Verification items for the finished model (mm, model axes). A direction names the side the tool comes from. Round coordinates to 2 decimals unless told otherwise and drop trailing zeros. Order: outer loops, then holes, each group sorted by start corner. A loop starts at its lowest first (then second) coordinate and runs counter-clockwise, first axis right, second up. Notation, with made-up numbers: M -27,32.25 L 11,32.25 A31 cw 11,57.25 Z; hole C 13,-22 d6. An arc over 180 degrees is marked long. Answer as a JSON object with one key per item and string values. Group by question number.
```python
from build123d import *

# Parameters (mm, degrees)
BOSS_EXTRUDE1_DEPTH     = 22.225
CUT_EXTRUDE1_DEPTH      = 15.875
CUT_EXTRUDE2_DEPTH      = 19.05
CUT_EXTRUDE3_DEPTH      = 19.05
CUT_EXTRUDE4_DEPTH      = 15.875
CUT_EXTRUDE5_DEPTH      = 1
CUT_EXTRUDE5_DEPTH_BACK = 45.45
CUT_EXTRUDE6_DEPTH      = 38.1
SKETCH9_R               = 4.75
CUT_EXTRUDE7_DEPTH      = 39.1
CUT_EXTRUDE7_DEPTH_BACK = 7.35
SKETCH10_R              = 5.08
CUT_EXTRUDE8_DEPTH      = 38.1
CUT_EXTRUDE8_DEPTH_BACK = 38.1
SKETCH14_R              = 5.08
CUT_EXTRUDE9_DEPTH      = 88.9


with BuildPart() as part:
    # Sketch1 → Boss-Extrude1 (new body, symmetric)
    with BuildSketch(Plane(origin=(0, 0, 0), x_dir=(1, 0, 0), z_dir=(0, 1, 0))):
        with BuildLine():
            Line((-27.139164257, 167.796683689), (23.215337255, 167.796683689))
            ThreePointArc((23.215337255, 167.796683689), (26.553400644, 166.414012561), (27.936071772, 163.075949172))
            Line((27.936071772, 163.075949172), (27.936071772, 117.442182176))
            Line((27.936071772, 117.442182176), (45.739076513, 99.639177435))
            ThreePointArc((45.739076513, 99.639177435), (52.653298853, 95.043473949), (60.717629895, 93.070271999))
            ThreePointArc((60.717629895, 93.070271999), (72.137749756, 94.950404711), (82.719311408, 99.639177435))
            ThreePointArc((82.719311408, 99.639177435), (99.088819495, 116.502407503), (106.691226482, 138.740499404))
            ThreePointArc((106.691226482, 138.740499404), (107.293250165, 146.399208048), (107.783318293, 154.065894676))
            ThreePointArc((107.783318293, 154.065894676), (108.340552038, 159.17256706), (108.853679748, 164.283859678))
            ThreePointArc((108.853679748, 164.283859678), (109.705429788, 167.387313473), (111.11535679, 170.2802375))
            ThreePointArc((111.11535679, 170.2802375), (113.620556723, 172.466184723), (116.845200472, 173.276162908))
            ThreePointArc((116.845200472, 173.276162908), (120.221594265, 172.465675408), (123.355683212, 170.970880603))
            ThreePointArc((123.355683212, 170.970880603), (128.265134652, 166.745027029), (132.181680011, 161.585451046))
            ThreePointArc((132.181680011, 161.585451046), (138.33428397, 146.199471549), (139.619453347, 129.678840803))
            ThreePointArc((139.619453347, 129.678840803), (136.39277719, 110.641651914), (129.659662699, 92.544934835))
            ThreePointArc((129.659662699, 92.544934835), (120.370646129, 69.036558024), (118.071361376, 43.864293549))
            ThreePointArc((118.071361376, 43.864293549), (122.222572829, 21.498106395), (129.659662699, 0))
            ThreePointArc((129.659662699, 0), (143.398814545, -36.155916163), (153.856513267, -73.393680656))
            ThreePointArc((153.856513267, -73.393680656), (158.275027292, -104.230564471), (157.301620264, -135.367185167))
            ThreePointArc((157.301620264, -135.367185167), (141.975051177, -176.275361149), (106.691226482, -202.032579498))
            ThreePointArc((106.691226482, -202.032579498), (54.098789107, -214.895017574), (0, -217.069367939))
            ThreePointArc((0, -217.069367939), (-54.004742533, -214.862710734), (-106.509687866, -202.032579498))
            ThreePointArc((-106.509687866, -202.032579498), (-141.094553776, -177.085698472), (-156.684587611, -137.394255213))
            ThreePointArc((-156.684587611, -137.394255213), (-153.316704731, -83.564621207), (-134.097306667, -33.170307338))
            ThreePointArc((-134.097306667, -33.170307338), (-118.452837363, -0.106574858), (-106.509687848, 34.466839857))
            ThreePointArc((-106.509687848, 34.466839857), (-104.952609842, 63.858154337), (-111.536110603, 92.544934857))
            ThreePointArc((-111.536110603, 92.544934857), (-124.146260861, 134.317832636), (-132.040568435, 177.232524599))
            ThreePointArc((-132.040568435, 177.232524599), (-132.180605283, 199.253892218), (-127.895077973, 220.854690763))
            ThreePointArc((-127.895077973, 220.854690763), (-123.677084376, 229.09027242), (-117.65146136, 236.112248103))
            ThreePointArc((-117.65146136, 236.112248103), (-112.585214143, 239.486704693), (-106.727388664, 241.141908245))
            ThreePointArc((-106.727388664, 241.141908245), (-101.521494245, 239.144724173), (-99.844107934, 233.82716307))
            Line((-99.844107934, 233.82716307), (-100.045578427, 207.171189317))
            ThreePointArc((-100.045578427, 207.171189317), (-94.278032432, 176.375383516), (-77.376792667, 149.993678943))
            ThreePointArc((-77.376792667, 149.993678943), (-61.159480832, 143.276248437), (-44.942168999, 149.993678947))
            Line((-44.942168999, 149.993678947), (-27.139164257, 167.796683689))
        make_face()
    extrude(amount=BOSS_EXTRUDE1_DEPTH, both=True)

    # Sketch2 → Cut-Extrude1 (cut)
    with BuildSketch(Plane(origin=(0, 22.225, 0), x_dir=(1, 0, 0), z_dir=(0, 1, 0))):
        with BuildLine():
            Line((-27.379271025, 93.081221646), (-27.379271025, 167.796683689))
            Line((-27.379271025, 167.796683689), (23.215337255, 167.796683689))
            ThreePointArc((23.215337255, 167.796683689), (26.728167178, 166.341621892), (28.183228975, 162.828791969))
            Line((28.183228975, 162.828791969), (28.183228975, 93.081221646))
            Line((28.183228975, 93.081221646), (-27.379271025, 93.081221646))
        make_face()
    extrude(amount=-CUT_EXTRUDE1_DEPTH, mode=Mode.SUBTRACT)

    # Sketch3 → Cut-Extrude2 (cut)
    with BuildSketch(Plane(origin=(0, 22.225, 0), x_dir=(1, 0, 0), z_dir=(0, 1, 0))):
        with BuildLine():
            Line((-40.873021025, -27.568778354), (-34.523021025, -27.568778354))
            Line((-34.523021025, -27.568778354), (-34.523021025, -21.218778354))
            ThreePointArc((-34.523021025, -21.218778354), (-32.663149086, -16.728650294), (-28.173021025, -14.868778354))
            Line((-28.173021025, -14.868778354), (28.976978975, -14.868778354))
            ThreePointArc((28.976978975, -14.868778354), (33.467107035, -16.728650294), (35.326978975, -21.218778354))
            Line((35.326978975, -21.218778354), (35.326978975, -27.568778354))
            Line((35.326978975, -27.568778354), (41.676978975, -27.568778354))
            ThreePointArc((41.676978975, -27.568778354), (43.473030199, -28.31272713), (44.216978975, -30.108778354))
            Line((44.216978975, -30.108778354), (44.216978975, -37.728778354))
            ThreePointArc((44.216978975, -37.728778354), (43.473030199, -39.524829578), (41.676978975, -40.268778354))
            Line((41.676978975, -40.268778354), (35.326978975, -40.268778354))
            Line((35.326978975, -40.268778354), (35.326978975, -46.618778354))
            ThreePointArc((35.326978975, -46.618778354), (33.467107035, -51.108906415), (28.976978975, -52.968778354))
            Line((28.976978975, -52.968778354), (-28.173021025, -52.968778354))
            ThreePointArc((-28.173021025, -52.968778354), (-32.663149086, -51.108906415), (-34.523021025, -46.618778354))
            Line((-34.523021025, -46.618778354), (-34.523021025, -40.268778354))
            Line((-34.523021025, -40.268778354), (-40.873021025, -40.268778354))
            ThreePointArc((-40.873021025, -40.268778354), (-42.66907225, -39.524829578), (-43.413021025, -37.728778354))
            Line((-43.413021025, -37.728778354), (-43.413021025, -30.108778354))
            ThreePointArc((-43.413021025, -30.108778354), (-42.66907225, -28.31272713), (-40.873021025, -27.568778354))
        make_face()
    extrude(amount=-CUT_EXTRUDE2_DEPTH, mode=Mode.SUBTRACT)

    # Sketch4 → Cut-Extrude3 (cut)
    with BuildSketch(Plane(origin=(0, 22.225, 0), x_dir=(1, 0, 0), z_dir=(0, 1, 0))):
        with BuildLine():
            Line((-40.873021025, 61.331221646), (-34.523021025, 61.331221646))
            Line((-34.523021025, 61.331221646), (-34.523021025, 67.681221646))
            ThreePointArc((-34.523021025, 67.681221646), (-32.663149086, 72.171349706), (-28.173021025, 74.031221646))
            Line((-28.173021025, 74.031221646), (28.976978975, 74.031221646))
            ThreePointArc((28.976978975, 74.031221646), (33.467107035, 72.171349706), (35.326978975, 67.681221646))
            Line((35.326978975, 67.681221646), (35.326978975, 61.331221646))
            Line((35.326978975, 61.331221646), (41.676978975, 61.331221646))
            ThreePointArc((41.676978975, 61.331221646), (43.473030199, 60.58727287), (44.216978975, 58.791221646))
            Line((44.216978975, 58.791221646), (44.216978975, 51.171221646))
            ThreePointArc((44.216978975, 51.171221646), (43.473030199, 49.375170422), (41.676978975, 48.631221646))
            Line((41.676978975, 48.631221646), (35.326978975, 48.631221646))
            Line((35.326978975, 48.631221646), (35.326978975, 42.281221646))
            ThreePointArc((35.326978975, 42.281221646), (33.467107035, 37.791093585), (28.976978975, 35.931221646))
            Line((28.976978975, 35.931221646), (-28.173021025, 35.931221646))
            ThreePointArc((-28.173021025, 35.931221646), (-32.663149086, 37.791093585), (-34.523021025, 42.281221646))
            Line((-34.523021025, 42.281221646), (-34.523021025, 48.631221646))
            Line((-34.523021025, 48.631221646), (-40.873021025, 48.631221646))
            ThreePointArc((-40.873021025, 48.631221646), (-42.66907225, 49.375170422), (-43.413021025, 51.171221646))
            Line((-43.413021025, 51.171221646), (-43.413021025, 58.791221646))
            ThreePointArc((-43.413021025, 58.791221646), (-42.66907225, 60.58727287), (-40.873021025, 61.331221646))
        make_face()
    extrude(amount=-CUT_EXTRUDE3_DEPTH, mode=Mode.SUBTRACT)

    # Sketch5 → Cut-Extrude4 (cut)
    with BuildSketch(Plane.XZ.offset(22.225)):
        with BuildLine():
            Line((-36.295157608, 111.718978354), (-36.295157608, -0.295021646))
            ThreePointArc((-36.295157608, -0.295021646), (-34.435285668, -4.785149706), (-29.945157608, -6.645021646))
            Line((-29.945157608, -6.645021646), (36.729842392, -6.645021646))
            ThreePointArc((36.729842392, -6.645021646), (41.219970453, -4.785149706), (43.079842392, -0.295021646))
            Line((43.079842392, -0.295021646), (43.079842392, 111.718978354))
            ThreePointArc((43.079842392, 111.718978354), (41.219970453, 116.209106415), (36.729842392, 118.068978354))
            Line((36.729842392, 118.068978354), (-29.945157608, 118.068978354))
            ThreePointArc((-29.945157608, 118.068978354), (-34.435285668, 116.209106415), (-36.295157608, 111.718978354))
        make_face()
    extrude(amount=-CUT_EXTRUDE4_DEPTH, mode=Mode.SUBTRACT)

    # Sketch6 → Cut-Extrude5 (cut, two sides)
    with BuildSketch(Plane.XZ.offset(22.225)) as cut_extrude5_sk:
        with BuildLine():
            Line((-29.945157608, 110.118778354), (36.729842392, 110.118778354))
            ThreePointArc((36.729842392, 110.118778354), (41.219970453, 108.258906415), (43.079842392, 103.768778354))
            Line((43.079842392, 103.768778354), (43.079842392, 99.018978354))
            ThreePointArc((43.079842392, 99.018978354), (41.219970453, 94.528850294), (36.729842392, 92.668978354))
            Line((36.729842392, 92.668978354), (-29.945157608, 92.668978354))
            ThreePointArc((-29.945157608, 92.668978354), (-34.435285668, 94.528850294), (-36.295157608, 99.018978354))
            Line((-36.295157608, 99.018978354), (-36.295157608, 103.768778354))
            ThreePointArc((-36.295157608, 103.768778354), (-34.435285668, 108.258906415), (-29.945157608, 110.118778354))
        make_face()
    extrude(amount=CUT_EXTRUDE5_DEPTH, mode=Mode.SUBTRACT)
    extrude(cut_extrude5_sk.sketch, amount=-CUT_EXTRUDE5_DEPTH_BACK, mode=Mode.SUBTRACT)

    # Sketch7 → Cut-Extrude6 (cut)
    with BuildSketch(Plane.XZ.offset(22.225)):
        with BuildLine():
            Line((63.367094077, -12.151361373), (108.743204002, 103.892460729))
            ThreePointArc((108.743204002, 103.892460729), (125.196118422, 111.095349531), (132.399007223, 94.642435111))
            Line((132.399007223, 94.642435111), (87.022897298, -21.401386992))
            ThreePointArc((87.022897298, -21.401386992), (70.569982878, -28.604275793), (63.367094077, -12.151361373))
        make_face()
    extrude(amount=-CUT_EXTRUDE6_DEPTH, mode=Mode.SUBTRACT)

    # Sketch9 → Cut-Extrude7 (cut, two sides)
    with BuildSketch(Plane.XZ.offset(-15.875)) as cut_extrude7_sk:
        with Locations((85.754227465, 10.292205969)):
            Circle(SKETCH9_R)
        with Locations((97.267975655, 39.880989361)):
            Circle(SKETCH9_R)
        with Locations((117.992722398, 93.140799466)):
            Circle(SKETCH9_R)
    extrude(amount=CUT_EXTRUDE7_DEPTH, mode=Mode.SUBTRACT)
    extrude(cut_extrude7_sk.sketch, amount=-CUT_EXTRUDE7_DEPTH_BACK, mode=Mode.SUBTRACT)

    # Sketch10 → Cut-Extrude8 (cut, two sides)
    with BuildSketch(Plane.XY) as cut_extrude8_sk:
        with Locations((-16.812366699, 12.116016476)):
            Circle(SKETCH10_R)
    extrude(amount=CUT_EXTRUDE8_DEPTH, mode=Mode.SUBTRACT)
    extrude(cut_extrude8_sk.sketch, amount=-CUT_EXTRUDE8_DEPTH_BACK, mode=Mode.SUBTRACT)

    # Sketch14 → Cut-Extrude9 (cut)
    with BuildSketch(Plane(origin=(44.388567954, 0, 22.168329827), x_dir=(0.446795069, 0, -0.894636332), z_dir=(0.894636332, 0, 0.446795069))):
        with Locations((-30.324577812, 12.371154411)):
            Circle(SKETCH14_R)
    extrude(amount=CUT_EXTRUDE9_DEPTH, mode=Mode.SUBTRACT)


solid = part.part
```
Q1. Cross-section at B-B, the plane x = -51. Record the cut outline in (y, z) (3 decimals).
Q2. Tool access check on faces 1 (the face through (-2, -8, -167.797)), 2 (the face through (1, 13, 52.969)), 3 (the face through (-118.647, 0.311, 0.581)). Record the directions out of +Z, -Z, +X, -X, +Y, -Y that give a thin tool (end or side, any length) a straight path to the whole face; none if there is none.
Q3. Thickness scan on line 1 (Z direction, x = 14, y = 3.5); line 2 (X direction, y = -17.5, z = 66.5); line 3 (Z direction, x = 38, y = 11). Record the ranges inside material, lowest first. Write a range as from..to.
Q4. Gauge pin test, flat ends, axial feed: pin 1 Ø1.9 at (y, z) = (15, -46.5) entering from +X; pin 2 Ø7 at (y, z) = (15.5, -46) entering from -X; pin 3 Ø5 at (x, y) = (-30.5, 4.5) entering from -Z; pin 4 Ø7.5 at (x, z) = (117.99, 93.14) entering from +Y. Record the tip position at first contact, or that the pin passes through.
Q5. Release check for a two-part mould opening along Z. For faces 4 (the face through (92.523, 19.006, 40.09)), 5 (the face through (68.377, 15.804, 72.229)), 6 (the face through (1, 6.35, -131)), 7 (the face through (71.982, 0.311, -94.904)) record: released by +Z, released by -Z, zero draft, split by the parting line, or undercut.
Q6. Cross-section at C-C, the plane y = -11. Give the number of separate pieces and of enclosed holes in the cut face, then the cut area to 3 significant figures.
Q7. Cross-section at D-D, the plane z = 149. Record the cut outline in (x, y) (3 decimals).
Q8. Cross-section at A-A, the plane z = -123.5. Record the cut outline in (x, y) (3 decimals), then the cut area to 3 significant figures.
Conclusion:
{
 "1": {"outline": "M -22.225,-145.649 L 22.225,-145.649 L 22.225,215.27 L -22.225,215.27 Z"},
 "2": {"face 1": "-Z, +Y, -Y", "face 2": "+Y", "face 3": "-X, +Y, -Y"},
 "3": {"line 1": "-167.8..-74.03, -35.93..14.87, 52.97..92.67, 110.12..217.54", "line 2": "-148.73..-36.3, 43.08..94.12, 121.39..152.19", "line 3": "-107.38..-61.33, -48.63..27.57, 40.27..47.41, 58.34..92.8, 109.99..216.68"},
 "4": {"pin 1": "x = 118", "pin 2": "x = -105.26", "pin 3": "z = -166.94", "pin 4": "through"},
 "5": {"face 4": "undercut", "face 5": "undercut", "face 6": "zero draft", "face 7": "released by -Z"},
 "6": {"separate pieces": "1", "enclosed holes": "2", "area": "84,600 mm2"},
 "7": {"outline": "M -154.736,-22.225 L 155.125,-22.225 L 155.125,22.225 L -154.736,22.225 Z"},
 "8": {"outline": "M -121.363,-22.225 L 27.936,-22.225 L 27.936,6.35 L -27.379,6.35 L -27.379,22.225 L -121.363,22.225 Z; M 102.702,-22.225 L 138.975,-22.225 L 138.975,22.225 L 102.702,22.225 Z", "area": "7,370 mm2"}
}
